Check sheet for the modelled part. Datum: model origin and axes. Units: mm. Round coordinates to 2 decimals unless told otherwise and drop trailing zeros. Order: outer loops, then holes, each group sorted by start corner. A loop starts at its lowest first (then second) coordinate and runs counter-clockwise, first axis right, second up. Notation, with made-up numbers: (10.5, 25) -> (54.5, 25) arc R10 cw to (54.5, 38) -> close; hole circle Ø5 at (-12, 11.25). An arc over 180 degrees is marked (long way). Use CSV: the item, a comma, the result in double quotes.
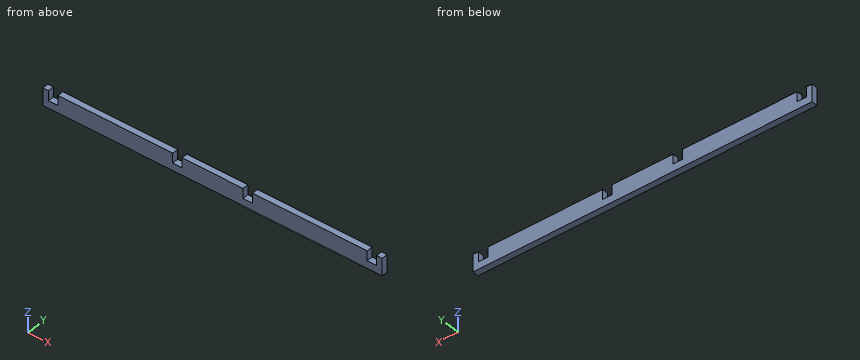
```python
from build123d import *

# Parameters (mm, degrees)
F1_DEPTH = 12


# Not quite as in the source:
# - a feature names something its author has since deleted; it is built from what else it names


with BuildPart() as f1:
    # F0 (on Front) → F1 (new body)
    with BuildSketch(Plane.XZ):
        Polygon((0, 35), (0, 0), (680, 0), (680, 35), (669, 35), (669, 15), (650, 15), (650, 35), (420, 35), (420, 15), (401, 15), (401, 35), (279, 35), (279, 15), (260, 15), (260, 35), (30, 35), (30, 15), (11, 15), (11, 35), align=None)
    extrude(amount=F1_DEPTH)


solid = f1.part
```
Q1. Sectioned sample at B-B, the plane y = -3. Enter the section's corners in (x, z).
Result sheet:
outline,"(0, 0) -> (680, 0) -> (680, 35) -> (669, 35) -> (669, 15) -> (650, 15) -> (650, 35) -> (420, 35) -> (420, 15) -> (401, 15) -> (401, 35) -> (279, 35) -> (279, 15) -> (260, 15) -> (260, 35) -> (30, 35) -> (30, 15) -> (11, 15) -> (11, 35) -> (0, 35) -> close"
Q2. Sectioned sample at A-A, the plane z = 21. Enter the section's corners in (x, y).
Result sheet:
outline,"(0, -12) -> (11, -12) -> (11, 0) -> (0, 0) -> close; (30, -12) -> (260, -12) -> (260, 0) -> (30, 0) -> close; (279, -12) -> (401, -12) -> (401, 0) -> (279, 0) -> close; (420, -12) -> (650, -12) -> (650, 0) -> (420, 0) -> close; (669, -12) -> (680, -12) -> (680, 0) -> (669, 0) -> close"
Q3. Scan lines: L1, parallel to X at y = -2.75, z = 25; L2, parallel to Z at x = 418, y = -2.25. Record each from-to range of solid material in increasing order.
Result sheet:
L1,"x = 0 to 11, 30 to 260, 279 to 401, 420 to 650, 669 to 680"
L2,"z = 0 to 15"
Q4. Go/stop test with a flat-tipped pin: pin 1 (3.5 mm diameter, centred on x = 25, y = -8, fed in from +Z). Record where the tip stops, or that it passes through.
Result sheet:
pin 1,"stops at z = 15"
